Part model, mm, in its own coordinate system. A direction names the side the tool comes from. Coordinates: 2 decimals unless noted, no trailing zeros. Loops run counter-clockwise (first coordinate to the right, second up) from the corner with the lowest first, then second, coordinate; pieces in that order, holes last. Notation, with made-up numbers: (49.25, 16.25) - (91.25, 16.25) arc R30 ccw to (91.25, 45.25) - close; hole circle Ø5 at (13.5, 59.25). An arc over 180 degrees is marked (long way). Use a Markdown table: item, result. Add a question column.
1. Band-saw the part on B-B, the plane x = 13.75. Give the cut face in (y, z).
2. Band-saw the part on A-A, the plane y = 35.5. Give the cut face in (x, z), plus the area to 3 significant figures.
3. Band-saw the part on D-D, the plane x = 5.75. Give the cut face in (y, z).
4. Wall check: probe 1 along Z at (x, y) = (3.5, -2); probe 2 along Y at (x, z) = (3.5, -0.5); probe 3 along Z at (x, y) = (2, 28). Give the ranges that are in metal, low to high. Write a range as [from, to].
5. Pull direction Y, two halves, no side cores. Call faces 5 (the cylindrical face through (7.64, 13.75, -5.54)), 6 (the cylindrical face through (7.605, 22.188, -6.495)), 7 (the flat face through (7, -5.21, -6)), 8 (the flat face through (4, 35, 10.934)): pulls with the +Y half, pulls with the -Y half, needs draft (parallel to the pull), parting line crosses it, or undercut.
6. 3-axis set-ups, long thin cutter, end or side, ignore diameter. For faces 1 (the flat face through (0, 21, 2)), 2 (the cylindrical face through (7.57, 45.89, 9.46)), 3 (the flat face through (7, 22.79, 2)), 4 (the flat face through (4, 7, -4.066)): which of +Z, -Z, +X, -X, +Y, -Y reach the whole face in a straight line?
7. Drop flat-ended pins along their axis: pin 1 (4 mm diameter, centred on x = 3, z = 1, fed in from +Y); pin 2 (8 mm diameter, centred on x = 12.5, z = 6, fed in from -Y). Give the stop position or say it passes through.
8. Band-saw the part on C-C, the plane z = -6. Give the cut face in (x, y).
Autodesk Inventor part; units mm, degrees
ref_plane "YZ Plane" through (0, 0, 0) normal (1, 0, 0) x (0, 1, 0)
ref_plane "XZ Plane" through (0, 0, 0) normal (0, 1, 0) x (-1, 0, 0)
ref_plane "XY Plane" through (0, 0, 0) normal (0, 0, 1) x (1, 0, 0)
sketch "Sketch1" plane through (0, 0, 0) normal (1, 0, 0) x (0, 1, 0)
  line L0 (47.7895, 7.9342) -> (22.7895, 7.9342)
  line L1 (22.7895, 7.9342) -> (22.7895, -7.0658)
  line L2 (22.7895, -7.0658) -> (-5.2105, -7.0658)
  line L3 (-5.2105, -7.0658) -> (-5.2105, -4.0658)
  line L4 (-5.2105, -4.0658) -> (19.7895, -4.0658)
  line L5 (19.7895, -4.0658) -> (19.7895, 10.9342)
  line L6 (19.7895, 10.9342) -> (47.7895, 10.9342)
  line L7 (47.7895, 10.9342) -> (47.7895, 7.9342)
  point P0 (0, 0)
  dimension "d0" = 3
  dimension "d1" = 3
  dimension "d2" = 3
  dimension "d3" = 15
  dimension "d4" = 25
  dimension "d5" = 25
extrude "Extrusion1" add sketch "Sketch1" along normal blind 15
fillet "Fillet1" radius 2 2 edges at (7.5, 22.7895, -7.0658) (7.5, 19.7895, 10.9342)
sketch "Sketch2" plane through (0, 47.7895, 10.9342) normal (0, 0, 1) x (1, 0, 0)
  arc A0 (10.6, -5) -> (4.4, -5) centre (7.5, -5) ccw
  line L0 (0, 0) -> (15, 0)
  arc A1 (4.4, -15) -> (10.6, -15) centre (7.5, -15) ccw
  line L1 (4.4, -15) -> (4.4, -5)
  line L2 (10.6, -5) -> (10.6, -15)
  line L3 (15, 0) -> (15, -26)
  arc A2 (10.6737, -37.1406) -> (4.4737, -37.1406) centre (7.5737, -37.1406) ccw
  line L4 (16.7377, 8.0467) -> (15.0737, 2.8292)
  arc A3 (4.4737, -47.1406) -> (10.6737, -47.1406) centre (7.5737, -47.1406) ccw
  line L5 (4.4737, -47.1406) -> (4.4737, -37.1406)
  line L6 (10.6737, -37.1406) -> (10.6737, -47.1406)
  line L7 (15.0737, 2.8292) -> (15.0737, -23.1708)
  point P0 (0, -47.7895)
  dimension "d9" = 6.2
  dimension "d10" = 5
  dimension "d11" = 6.2
  dimension "d12" = 10
  dimension "d13" = 7.5
  dimension "d15" = 7.5
  dimension "d16" = 6.2
  dimension "d17" = 5
  dimension "d18" = 6.2
  dimension "d19" = 10
  dimension "d20" = 7.5
  dimension "d21" = 7.5
extrude "Extrusion2" cut sketch "Sketch2" against normal blind 20
properties part number "Side holding bracket"
Geometry check:
| question | item | result |
|---|---|---|
| 1 | outline | (-5.21, -7.07) - (20.79, -7.07) arc R2 ccw to (22.79, -5.07) - (22.79, 7.93) - (47.79, 7.93) - (47.79, 10.93) - (21.79, 10.93) arc R2 ccw to (19.79, 8.93) - (19.79, -4.07) - (-5.21, -4.07) - close |
| 2 | outline | (0, 7.93) - (4.4, 7.93) - (4.4, 10.93) - (0, 10.93) - close; (10.6, 7.93) - (15, 7.93) - (15, 10.93) - (10.6, 10.93) - close |
| 2 | area | 26.4 mm^2 |
| 3 | outline | (-5.21, -7.07) - (-1.86, -7.07) - (-1.86, -4.07) - (-5.21, -4.07) - close; (13.16, -7.07) - (20.79, -7.07) arc R2 ccw to (22.79, -5.07) - (22.79, 7.93) - (30.23, 7.93) - (30.23, 10.93) - (21.79, 10.93) arc R2 ccw to (19.79, 8.93) - (19.79, -4.07) - (13.16, -4.07) - close; (45.35, 7.93) - (47.79, 7.93) - (47.79, 10.93) - (45.35, 10.93) - close |
| 4 | probe 1 | z = [-7.07, -4.07] |
| 4 | probe 2 | y = [19.79, 22.79] |
| 4 | probe 3 | z = [7.93, 10.93] |
| 5 | face 5 | undercut |
| 5 | face 6 | pulls with the +Y half |
| 5 | face 7 | pulls with the -Y half |
| 5 | face 8 | needs draft |
| 6 | face 1 | +Z, -Z, -X, +Y, -Y |
| 6 | face 2 | +Z, -Z |
| 6 | face 3 | -Z, +X, -X, +Y |
| 6 | face 4 | +Z, +X, -X, -Y |
| 7 | pin 1 | stops at y = 22.79 |
| 7 | pin 2 | stops at y = 19.79 |
| 8 | outline | (0, -5.21) - (15, -5.21) - (15, 22.56) - (0, 22.56) - close; hole (4.47, 0.65) arc R3.1 ccw to (10.67, 0.65) - (10.67, 10.65) arc R3.1 ccw to (4.47, 10.65) - close |
